from build123d import *

# Parameters (mm, degrees)
SKETCH1_R             = 25
SKETCH1_W             = 37
SKETCH1_H             = 27
SKETCH1_W_2           = 35
SKETCH1_H_2           = 25
BOSS_EXTRUDE1_DEPTH   = 4
SKETCH1_3_W           = 35
SKETCH1_3_H           = 25
BOSS_EXTRUDE2_DEPTH   = 1
M2X0_4_TAPPED_HOLE1_D = 1.6


with BuildPart() as part:
    # Sketch1 → Boss-Extrude1 (new body)
    # profile 1 of 2: a face of its own
    with BuildSketch(Plane.XY):
        Circle(SKETCH1_R)
        Rectangle(SKETCH1_W, SKETCH1_H, mode=Mode.SUBTRACT)
    # profile 2 of 2: a face of its own
    with BuildSketch(Plane.XY):
        Rectangle(SKETCH1_W, SKETCH1_H)
        Rectangle(SKETCH1_W_2, SKETCH1_H_2, mode=Mode.SUBTRACT)
    extrude(amount=BOSS_EXTRUDE1_DEPTH)

    # Sketch1_3 → Boss-Extrude2 (add)
    with BuildSketch(Plane.XY):
        Rectangle(SKETCH1_3_W, SKETCH1_3_H)
    extrude(amount=BOSS_EXTRUDE2_DEPTH)

    # Sketch2 → Revolve1 (revolve)
    with BuildSketch(Plane(origin=(0, 0, 0), x_dir=(1, 0, 0), z_dir=(0, 1, 0)), mode=Mode.PRIVATE) as revolve1_sk:
        with BuildLine():
            Line((0, 6.5), (0, 0))
            Line((0, 0), (-6.5, 0))
            ThreePointArc((-6.5, 0), (-4.596194078, 4.596194078), (0, 6.5))
        make_face()
    revolve(revolve1_sk.sketch.rotate(Axis((0, 0, -15), (0, 0, 1)), 180), axis=Axis((0, 0, -15), (0, 0, 1)))

    # M2x0.4 Tapped Hole1 (through all)
    with Locations(Plane.XY.offset(4)):
        with Locations((-21, 0), (14, -16), (14, 16)):
            Hole(M2X0_4_TAPPED_HOLE1_D / 2)


solid = part.part
Here's how the part is built. I have some questions about the finished solid (model axes, mm). A direction names the side the tool comes from. Give positions to 0.01 mm unless a question says otherwise; leave off trailing zeros. Order: outer loops, then holes, each group sorted by start corner. A loop starts at its lowest first (then second) coordinate and runs counter-clockwise, first axis right, second up. Notation, with made-up numbers: (45.25, 57) -> (58.25, 57) arc R19 cw to (58.25, 79) -> close; hole circle Ø4 at (29.5, 0). An arc over 180 degrees is marked (long way). One line per item, written item: value. Start each with the question number.
1. Imagine slicing it at A-A, the plane y = 0. List the corners of the cut face in (x, z) for me.
2. Imagine slicing it at B-B, the plane x = 0. List the corners of the cut face in (y, z) for me, plus the area to 3 significant figures.
3. We'd pull the mould along X, two halves only. Please class faces 1 (the face through (0, -12.5, 2)), 2 (the face through (23.846, 7.509, 1.972)), 3 (the face through (5, -5, 0)): released by +X, released by -X, zero draft, split by the parting line, or undercut.
4. Imagine slicing it at C-C, the plane z = 3.25. List the corners of the cut face in (x, y) for me, plus the area to 3 significant figures.
5. Will these pins go through, and if not, where does the flat tip stop? pin 1 Ø3.5 at (y, z) = (5.5, 3) entering from +X; pin 2 Ø4 at (x, y) = (14, 11) entering from -Z; pin 3 Ø3.5 at (x, z) = (0, 2) entering from +Y; pin 4 Ø2 at (y, z) = (6, -5) entering from +X.
6. Imagine slicing it at D-D, the plane x = -21. List the corners of the cut face in (y, z) for me.
7. For faces 4 (the face through (0, 0, 1)), 5 (the face through (-20.41, 0.54, 1.97)), which set-ups out of +Z, -Z, +X, -X, +Y, -Y let a thin tool reach every point of the face, with its end or its side?
8. I need wall thicknesses on probe 1 along Y at (x, z) = (14, 2.3); probe 2 along Z at (x, y) = (-20.5, 7); probe 3 along Z at (x, y) = (2, -10). Which ranges of each line are inside material? Lowest first, please. Write a range as from..to.
Values follow:
1. outline: (-25, 0) -> (-21.8, 0) -> (-21.8, 4) -> (-25, 4) -> close; (-20.2, 0) -> (-6.5, 0) arc R6.5 ccw to (6.5, 0) -> (25, 0) -> (25, 4) -> (17.5, 4) -> (17.5, 1) -> (-17.5, 1) -> (-17.5, 4) -> (-20.2, 4) -> close
2. outline: (-25, 0) -> (-6.5, 0) arc R6.5 ccw to (6.5, 0) -> (25, 0) -> (25, 4) -> (12.5, 4) -> (12.5, 1) -> (-12.5, 1) -> (-12.5, 4) -> (-25, 4) -> close
2. area: 191 mm2
3. face 1: undercut
3. face 2: split by the parting line
3. face 3: zero draft
4. outline: circle Ø50 at (0, 0); hole circle Ø1.6 at (-21, 0); hole (-17.5, -12.5) -> (17.5, -12.5) -> (17.5, 12.5) -> (-17.5, 12.5) -> close; hole circle Ø1.6 at (14, -16); hole circle Ø1.6 at (14, 16)
4. area: 1,080 mm2
5. pin 1: stops at x = 24.72
5. pin 2: stops at z = 0
5. pin 3: stops at y = 25
5. pin 4: passes through
6. outline: (-13.56, 0) -> (-0.8, 0) -> (-0.8, 4) -> (-13.56, 4) -> close; (0.8, 0) -> (13.56, 0) -> (13.56, 4) -> (0.8, 4) -> close
7. face 4: +Z
7. face 5: +Z, -Z
8. probe 1: y = -20.71..-16.8, -15.2..-12.5, 12.5..15.2, 16.8..20.71
8. probe 2: z = 0..4
8. probe 3: z = 0..1
